```python
from build123d import *

# Parameters (mm, degrees)
PAD010_DEPTH      = 15
PAD010_DEPTH_BACK = 15
SKETCH020_R       = 2.2
POCKET004_DEPTH   = 5
FILLET009_R       = 1


with BuildPart() as part:
    # Sketch019 → Pad010 (new body, two sides)
    with BuildSketch(Plane.YZ) as pad010_sk:
        with BuildLine():
            Line((-49.572759, 0), (-49.572759, -3))
            Line((-49.572759, -3), (-34.572759, -3))
            ThreePointArc((-34.572759, -3), (-32.672925, -13.506221), (-27.214047, -22.681771))
            Line((-38.53469, -32.522656), (-27.214047, -22.681771))
            Line((-38.53469, -32.522656), (-36.566513, -34.786785))
            Line((-36.566513, -34.786785), (0, -3))
            Line((0, -3), (15, -3))
            Line((15, 0), (15, -3))
            Line((15, 0), (-49.572759, 0))
        make_face()
        with BuildLine():
            Line((-4.572759, -3), (-24.949918, -20.713594))
            ThreePointArc((-31.572759, -3), (-29.862908, -12.455599), (-24.949918, -20.713594))
            Line((-31.572759, -3), (-4.572759, -3))
        make_face(mode=Mode.SUBTRACT)
    extrude(amount=-PAD010_DEPTH)
    extrude(pad010_sk.sketch, amount=PAD010_DEPTH_BACK)

    # Sketch020 → Pocket004 (cut)
    with BuildSketch(Plane.XY):
        with Locations((0, 9.8)):
            Circle(SKETCH020_R)
        with Locations((0, -44.372759)):
            Circle(SKETCH020_R)
    extrude(amount=-POCKET004_DEPTH, mode=Mode.SUBTRACT)

    # Fillet009
    fillet009_edges = [part.edges().sort_by_distance(p)[0] for p in [
        (0, -49.572759, 0),
        (0, -49.572759, -3),
        (0, -34.572759, -3),
        (0, -27.214047, -22.681771),
        (0, -38.53469, -32.522656),
        (0, -36.566513, -34.786785),
        (0, -31.572759, -3),
        (0, -4.572759, -3),
        (0, -24.949918, -20.713594),
        (0, 15, 0),
        (0, 15, -3),
        (0, 0, -3),
    ]]
    fillet(fillet009_edges, radius=FILLET009_R)


solid = part.part
```
Could you check a few things on this model? Use its own coordinates, in mm. A direction names the side the tool comes from. Coordinates: 2 decimals unless noted, no trailing zeros. Loops run counter-clockwise (first coordinate to the right, second up) from the corner with the lowest first, then second, coordinate; pieces in that order, holes last. Notation, with made-up numbers: M 5,-20 L 55,-20 A25 ccw 55,-3 Z; hole C -15.5,-7.75 d4. An arc over 180 degrees is marked long. Put each result on its own line as item: value. Start each with the question number.
(1) Suppose I cut it at A-A on y = 9.8. Please give me the cut outline in (x, z).
(2) Will these pins go through, and if not, where does the flat tip stop? P1, Ø5, axis at x = -9, z = -29.5, coming from the +Y side; P2, Ø2, axis at x = -11, z = -24, coming from the -Y side; P3, Ø10, axis at x = -5.5, y = -17, coming from the -Z side.
(3) Suppose I cut it at B-B on x = 0. Count the separate pieces of the cut face and the enclosed holes in it, then the cut area to 3 significant figures.
(4) Suppose I cut it at C-C on x = 12.25. Please give me the cut outline in (y, z), then the cut area to 3 significant figures.
(5) Suppose I cut it at D-D on z = -19. Please give me the cut outline in (x, y).
(6) Thinking about a two-plate mould opening in X: for faces 1 (the face through (-0.48, -46.52, -1.48)), 2 (the face through (-15, -17, -15)), 3 (the face through (0.21, -6.32, -3.63)), which applies, pulls with the +X half, pulls with the -X half, needs draft (parallel to the pull), parting line crosses it, or undercut?
(7) I need wall thicknesses on line 1 (Y direction, x = 0, z = -1.15); line 2 (Y direction, x = 0, z = -2.25); line 3 (Z direction, x = -8, y = -29). Which ranges of each line are inside material? Lowest first, please. Write a range as from..to.
(8) For faces 4 (the face through (-0.477, 7.652, -1.479)), 5 (the face through (-0.21, -32.94, -27.66)), 6 (the face through (0, 7, -3)), 7 (the face through (-0.21, -36.527, -34.374)), 8 (the face through (-0.21, -15.26, -12.29)), which set-ups out of +Z, -Z, +X, -X, +Y, -Y let a thin tool reach every point of the face, with its end or its side?
Solutions:
1. outline: M -15,-3 L -2.2,-3 L -2.2,0 L -15,0 Z; M 2.2,-3 L 15,-3 L 15,0 L 2.2,0 Z
2. P1: stops at y = -27.61
2. P2: stops at y = -29.88
2. P3: stops at z = -22.12
3. separate pieces: 3
3. enclosed holes: 1
3. area: 370 mm2
4. outline: M -49.57,-2 A1 ccw -48.57,-3 L -35.56,-3 A1 cw -34.56,-3.97 A30 ccw -27.84,-21.94 A1 cw -27.96,-23.33 L -37.78,-31.87 A1 ccw -37.88,-33.28 L -37.22,-34.03 A1 ccw -35.81,-34.13 L -0.28,-3.25 A1 cw 0.37,-3 L 14,-3 A1 ccw 15,-2 L 15,-1 A1 ccw 14,0 L -48.57,0 A1 ccw -49.57,-1 Z; hole M -31.55,-4.04 A27 ccw -25.62,-19.92 A1 ccw -24.18,-20.04 L -6.59,-4.75 A1 ccw -7.25,-3 L -30.55,-3 A1 ccw Z
4. area: 396 mm2
5. outline: M -15,-29.95 L 15,-29.95 L 15,-26.32 L -15,-26.32 Z; M -15,-22.98 L 15,-22.98 L 15,-18.41 L -15,-18.41 Z
6. face 1: undercut
6. face 2: pulls with the -X half
6. face 3: needs draft
7. line 1: y = -49.57..-46.57, -42.17..7.6, 12..15
7. line 2: y = -49.54..-46.57, -42.17..7.6, 12..14.97
7. line 3: z = -28.21..-24.23, -20.42..-14.5, -3..0
8. face 4: +Z, -Z
8. face 5: +X, -X, -Y
8. face 6: -Z, +X, -X, +Y
8. face 7: -Z, +X, -X
8. face 8: +X, -X
